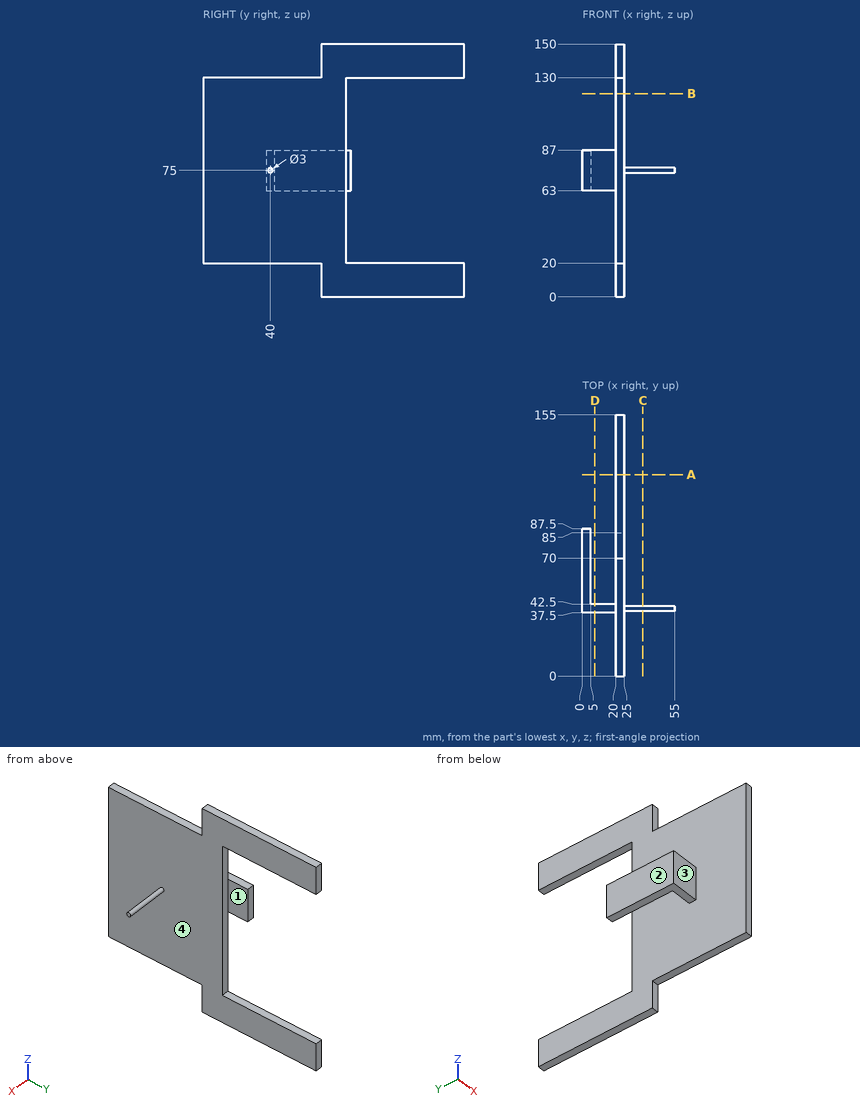
Could you check a few things on this drawing? It's one solid part, dimensions in mm from its lowest x, y, z. Give positions to 0.01 mm unless a question says otherwise; leave off trailing zeros. Order: outer loops, then holes, each group sorted by start corner. A loop starts at its lowest first (then second) coordinate and runs counter-clockwise, first axis right, second up. Notation, with made-up numbers: (-18, 76) - (35, 76) arc R27 ccw to (35, 105) - close; hole circle Ø3 at (67.25, 79.5). An arc over 180 degrees is marked (long way). One line per item, written item: value. Start each with the question number.
1. Imagine slicing it at C-C on x = 36. List the corners of the cut face in (y, z) for me.
2. Imagine slicing it at A-A on y = 119.5. List the corners of the cut face in (x, z) for me, plus the area to 3 significant figures.
3. If I drill on probe 1 along Z at (x, y) = (20.5, 111); probe 2 along Z at (x, y) = (7, 38); probe 3 along Z at (x, y) = (22, 51), over which ranges is the centre line in solid material (lowest first)?
4. Imagine slicing it at B-B on z = 120.5. List the corners of the cut face in (x, y) for me.
5. Thinking about a two-plate mould opening in X: for the marked faces 1, 2, 3 and 4, which applies, +X half, -X half, draft (parallel to the pull), parting line (faces both ways), or undercut?
6. Imagine slicing it at D-D on x = 7.5. List the corners of the cut face in (y, z) for me.
7. For P1, Ø1.5, axis at x = 22.5, z = 135.5, coming from the -Y side; P2, Ø2.5, axis at x = 1.5, z = 79.5, coming from the +Y side; P3, Ø5.5, axis at x = 22, y = 45, coming from the +Z side, each with a flat end and sliding along its axis, tell me the tip position at first contact or that it passes through.
Values:
1. outline: circle Ø3 at (40, 75)
2. outline: (20, 0) - (25, 0) - (25, 20) - (20, 20) - close; (20, 130) - (25, 130) - (25, 150) - (20, 150) - close
2. area: 200 mm²
3. probe 1: 0 to 20, 130 to 150
3. probe 2: 63 to 87
3. probe 3: 20 to 130
4. outline: (20, 0) - (25, 0) - (25, 85) - (20, 85) - close
5. face 1: undercut
5. face 2: -X half
5. face 3: draft
5. face 4: +X half
6. outline: (37.5, 63) - (42.5, 63) - (42.5, 87) - (37.5, 87) - close
7. P1: y = 70
7. P2: y = 87.5
7. P3: z = 130
